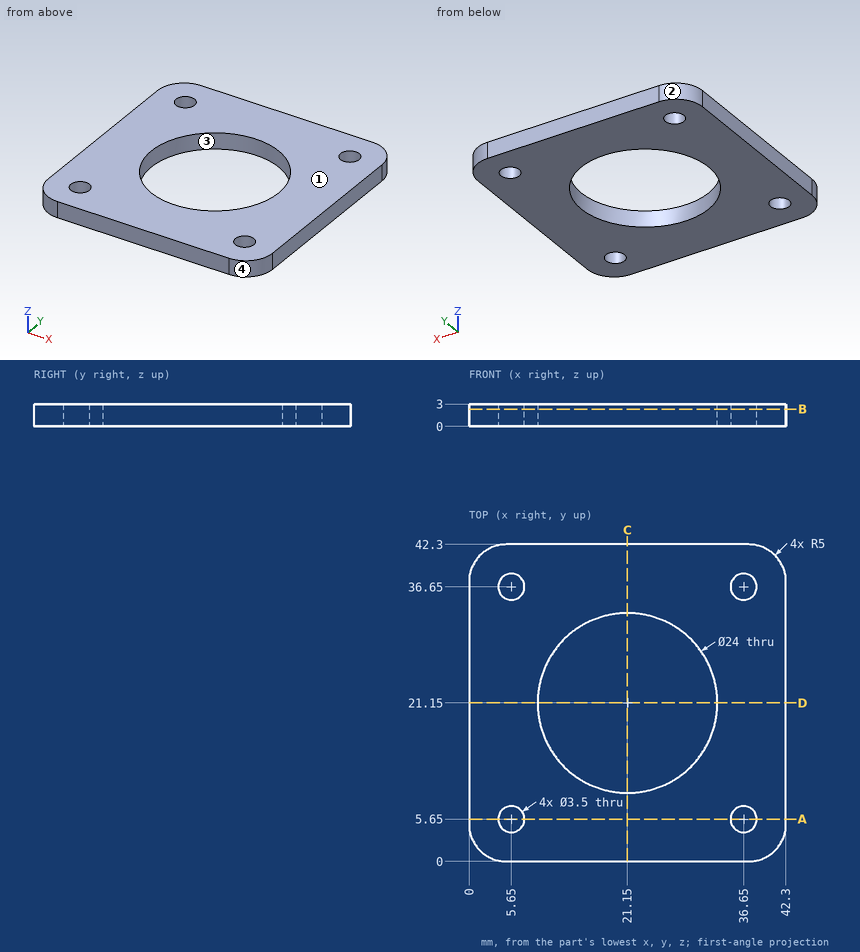
The figure shows three views and two pictorial views of one solid part (mm, origin at its lowest corner). Answer the questions. Give positions to 0.01 mm unless a question says otherwise; leave off trailing zeros. Write each loop counter-clockwise with the first axis right and the second up, starting at its lowest first coordinate (ties: lowest second). Pieces come first, ordered by that corner, then holes. Notation, with made-up numbers: (-33, -7.75) -> (17, -7.75) arc R18 ccw to (17, 21.25) -> close; hole circle Ø9 at (50, 1). An arc over 180 degrees is marked (long way). Use one line per item in the form item = value.
1) Section B-B on z = 2.3 is taken. Write down the section's boundary in (x, y).
Result:
outline = (0, 5) arc R5 ccw to (5, 0) -> (37.3, 0) arc R5 ccw to (42.3, 5) -> (42.3, 37.3) arc R5 ccw to (37.3, 42.3) -> (5, 42.3) arc R5 ccw to (0, 37.3) -> close; hole circle Ø3.5 at (5.65, 5.65); hole circle Ø3.5 at (5.65, 36.65); hole circle Ø24 at (21.15, 21.15); hole circle Ø3.5 at (36.65, 5.65); hole circle Ø3.5 at (36.65, 36.65)
2) For a pull along X with two mould halves and no side action, classify the marked faces 1, 2, 3 and 4 as +X half, -X half, draft (parallel to the pull), parting line (faces both ways), or undercut.
Result:
face_1 = draft
face_2 = -X half
face_3 = undercut
face_4 = +X half
3) Section C-C on x = 21.15 is taken. Write down the section's boundary in (y, z), plus the area to 3 significant figures.
Result:
outline = (0, 0) -> (9.15, 0) -> (9.15, 3) -> (0, 3) -> close; (33.15, 0) -> (42.3, 0) -> (42.3, 3) -> (33.15, 3) -> close
area = 54.9 mm²
4) Straight lines are drawn through the part: probe 1 along Y at (x, z) = (5.65, 1.9); probe 2 along Y at (x, z) = (21.15, 2.15); probe 3 along Y at (x, z) = (7, 0.5). For each, find the intervals that lie inside material, in ascending order.
Result:
probe_1 = 0 to 3.9, 7.4 to 34.9, 38.4 to 42.3
probe_2 = 0 to 9.15, 33.15 to 42.3
probe_3 = 0 to 4.54, 6.76 to 35.54, 37.76 to 42.3
5) Section A-A on y = 5.65 is taken. Write down the section's boundary in (x, z).
Result:
outline = (0, 0) -> (3.9, 0) -> (3.9, 3) -> (0, 3) -> close; (7.4, 0) -> (34.9, 0) -> (34.9, 3) -> (7.4, 3) -> close; (38.4, 0) -> (42.3, 0) -> (42.3, 3) -> (38.4, 3) -> close
